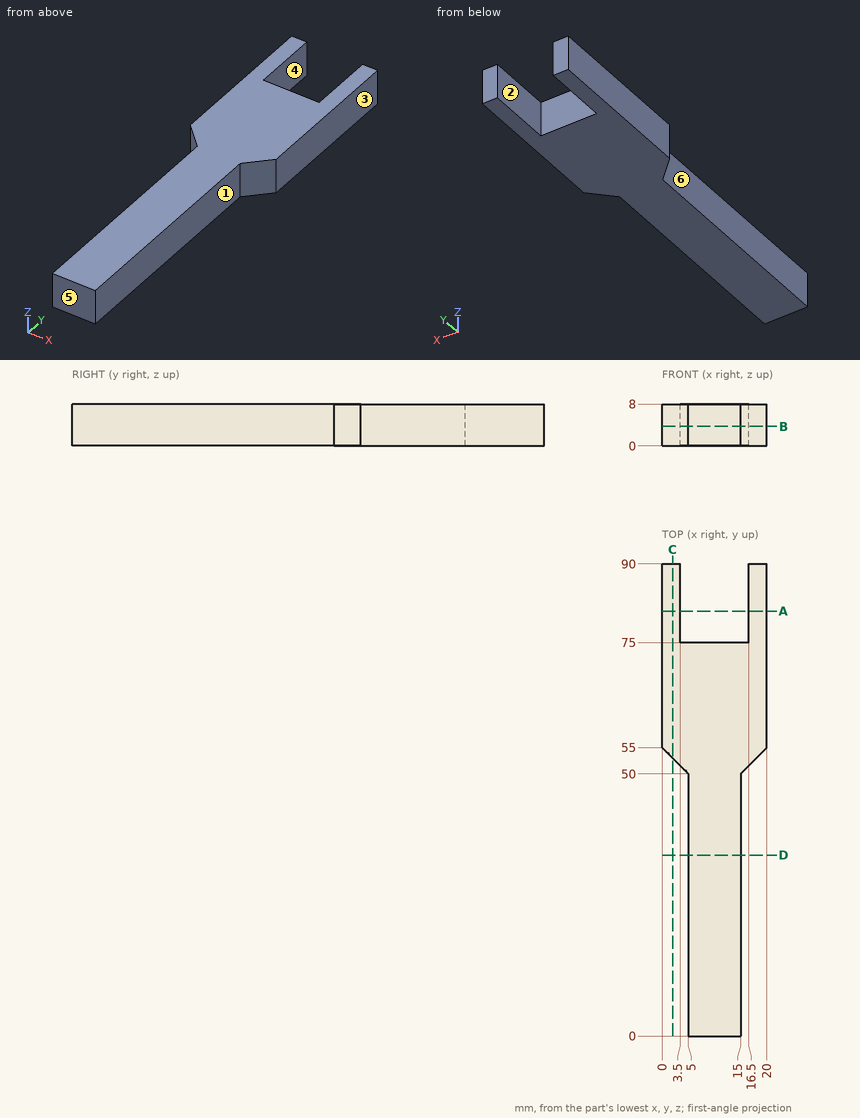
Here's the drawing with two shaded views (mm, measured from the low corner). I have some questions. A direction names the side the tool comes from. Round coordinates to 2 decimals unless told otherwise and drop trailing zeros. Write each loop counter-clockwise with the first axis right and the second up, starting at its lowest first coordinate (ties: lowest second). Pieces come first, ordered by that corner, then holes.
(1) If I drill on probe 1 along X at (y, z) = (43, 7.25); probe 2 along Y at (x, z) = (9.75, 7.5); probe 3 along Y at (x, z) = (4.75, 5), over which ranges is the centre line in solid material (lowest first)?
Findings below:
probe 1: x = 5 to 15
probe 2: y = 0 to 75
probe 3: y = 50.25 to 75
(2) Thinking about a two-plate mould opening in X: for the marked faces 4, 5 and 6, which applies, +X half, -X half, draft (parallel to the pull), parting line (faces both ways), or undercut?
Findings below:
face 4: undercut
face 5: draft
face 6: -X half
(3) Suppose I cut it at D-D on y = 34.5. Write out the boundary of the cut face in (x, z), and give its area (3 significant figures).
Findings below:
outline: (5, 0) - (15, 0) - (15, 8) - (5, 8) - close
area: 80.0 mm2
(4) Suppose I cut it at C-C on x = 2. Write out the boundary of the cut face in (y, z), and give its area (3 significant figures).
Findings below:
outline: (53, 0) - (90, 0) - (90, 8) - (53, 8) - close
area: 296 mm2
(5) Which directions (+Z, -Z, +X, -X, +Y, -Y) give clear straight access to the entire face, cutting with the end or side of a thin tool? Please do the marked faces 1, 2 and 3.
Findings below:
face 1: +Z, -Z, +X, -Y
face 2: +Z, -Z, +Y
face 3: +Z, -Z, +X, +Y, -Y
(6) For pin 1 (3 mm diameter, centred on y = 54, z = 3, fed in from +X); pin 2 (4 mm diameter, centred on x = 7, z = 4, fed in from +Y); pin 3 (4 mm diameter, centred on y = 24, z = 5, fed in from +X); pin 4 (4 mm diameter, centred on y = 37.5, z = 3, fed in from -X), each with a flat end and sliding along its axis, tell me the tip position at first contact or that it passes through.
Findings below:
pin 1: stops at x = 20
pin 2: stops at y = 75
pin 3: stops at x = 15
pin 4: stops at x = 5
(7) Suppose I cut it at A-A on y = 81. Write out the boundary of the cut face in (x, z), and give its area (3 significant figures).
Findings below:
outline: (0, 0) - (3.5, 0) - (3.5, 8) - (0, 8) - close; (16.5, 0) - (20, 0) - (20, 8) - (16.5, 8) - close
area: 56.0 mm2
(8) Suppose I cut it at B-B on z = 3.75. Write out the boundary of the cut face in (x, y).
Findings below:
outline: (0, 55) - (5, 50) - (5, 0) - (15, 0) - (15, 50) - (20, 55) - (20, 90) - (16.5, 90) - (16.5, 75) - (3.5, 75) - (3.5, 90) - (0, 90) - close
